The model under review builds one solid part; all positions refer to its coordinate system, in mm. A direction names the side the tool comes from. Round coordinates to 2 decimals unless told otherwise and drop trailing zeros. Loops run counter-clockwise (first coordinate to the right, second up) from the corner with the lowest first, then second, coordinate; pieces in that order, holes last. Notation, with made-up numbers: M -38,0 L -15,0 A17 cw -15,15 Z; hole C 52.25,-10.75 d2. An arc over 180 degrees is marked long. Answer as a JSON object with one key per item and string values. Group by question number.
Item 1: Consider section A-A (y = 20.5). Give the boundary of the cut face in (x, z), and give its area (3 significant figures).
Item 2: Consider section C-C (y = 10.75). Give the boundary of the cut face in (x, z), and give its area (3 significant figures).
Item 3: The part is to be moulded in two halves that separate along X. For faces 3 (the face through (-1, 23, 0)), 4 (the face through (19, 0, -7)), 5 (the face through (1, 23, 0)), 6 (the face through (19.394, 11.586, 12.365)), say which applies: +X half, -X half, draft (parallel to the pull), parting line (faces both ways), or undercut.
Item 4: Tool access review of faces 1 (the face through (0, 12, 0)), 2 (the face through (0, 25, 0)): name each direction out of +Z, -Z, +X, -X, +Y, -Y from which nothing blocks a thin tool from reaching the whole face with its end or side.
Item 5: To check wall thickness, follow line 1 (Z direction, x = -0.5, y = 16); line 2 (X direction, y = 11.9, z = 0); line 3 (Y direction, x = -1, z = 0). State the ranges of each line that lie inside material, in increasing order.
Item 6: Insertion check: P1, Ø1.3, axis at x = -2.5, z = -1.5, coming from the -Y side; P2, Ø8, axis at x = -11, y = 20, coming from the +Z side; P3, Ø5, axis at y = 15.5, z = -1.5, coming from the +X side. Each pin has a flat end and moves straight along its axis. Give the tip position at first contact, or say it passes through.
Item 7: Consider section B-B (y = 3.75). Give the boundary of the cut face in (x, z), and give its area (3 significant figures).
```python
from build123d import *

# Parameters (mm, degrees)
SKETCH1_R           = 23
BOSS_EXTRUDE1_DEPTH = 25
CUT_EXTRUDE1_DEPTH  = 23
SKETCH4_R           = 10
CUT_EXTRUDE2_DEPTH  = 12
CHAMFER1_SIZE       = 10
CHAMFER1_SIZE2      = 11.917535926
FILLET1_R           = 1.5
FILLET2_R           = 1


with BuildPart() as part:
    # Sketch1 → Boss-Extrude1 (new body)
    with BuildSketch(Plane(origin=(0, 0, 0), x_dir=(1, 0, 0), z_dir=(0, 1, 0))):
        with Locations(Location((0, 0, 0), (0, 0, 270))):
            Circle(SKETCH1_R)
    extrude(amount=BOSS_EXTRUDE1_DEPTH)

    # Sketch3 → Cut-Extrude1 (cut)
    with BuildSketch(Plane(origin=(0, 0, 0), x_dir=(-1, 0, 0), z_dir=(0, -1, 0))):
        with BuildLine():
            Line((-0.45, -3.067164815), (-0.45, 3.067164815))
            ThreePointArc((-0.45, 3.067164815), (-3.1, 0), (-0.45, -3.067164815))
        make_face()
        with BuildLine():
            ThreePointArc((3.1, 0), (2.345740821, 2.02669682), (0.45, 3.067164815))
            Line((0.45, 3.067164815), (0.45, -3.067164815))
            ThreePointArc((0.45, -3.067164815), (2.345740821, -2.02669682), (3.1, 0))
        make_face()
    extrude(amount=-CUT_EXTRUDE1_DEPTH, mode=Mode.SUBTRACT)

    # Sketch4 → Cut-Extrude2 (cut)
    with BuildSketch(Plane(origin=(0, 0, 0), x_dir=(-1, 0, 0), z_dir=(0, -1, 0))):
        with Locations(Location((0, 0, 0), (0, 0, 90))):
            Circle(SKETCH4_R)
    extrude(amount=-CUT_EXTRUDE2_DEPTH, mode=Mode.SUBTRACT)

    # Chamfer1
    chamfer1_edges = [part.edges().sort_by_distance(p)[0] for p in [
        (0, 0, 10),
    ]]
    chamfer1_side = [part.faces().sort_by_distance(p)[0] for p in [
        (0, 0, -22.349461761),
    ]]
    chamfer(chamfer1_edges, length=CHAMFER1_SIZE, length2=CHAMFER1_SIZE2, reference=chamfer1_side[0])

    # Fillet1
    fillet1_edges = [part.edges().sort_by_distance(p)[0] for p in [
        (0, 25, -23),
    ]]
    fillet(fillet1_edges, radius=FILLET1_R)

    # Sketch5 → Cut-Revolve1 (revolve, cut)
    with BuildSketch(Plane.XY):
        with BuildLine():
            Line((13, 25), (13, 23.5))
            ThreePointArc((13, 23.5), (14.60360392, 24.042792159), (16, 25))
            Line((16, 25), (13, 25))
        make_face()
    revolve(axis=Axis((13, 25, 0), (0, -1, 0)), mode=Mode.SUBTRACT)

    # Fillet2
    fillet2_edges = [part.edges().sort_by_distance(p)[0] for p in [
        (10, 25, 0),
    ]]
    fillet(fillet2_edges, radius=FILLET2_R)


solid = part.part
```
Geometry results:
{
 "1": {"outline": "C 0,0 d46; hole M -0.45,-3.07 L -0.45,3.07 A3.1 ccw Z; hole M 0.45,-3.07 A3.1 ccw 0.45,3.07 Z", "area": "1,640 mm^2"},
 "2": {"outline": "C 0,0 d46; hole C 0,0 d21.96", "area": "1,280 mm^2"},
 "3": {"face 3": "undercut", "face 4": "draft", "face 5": "undercut", "face 6": "parting line"},
 "4": {"face 1": "-Y", "face 2": "+Z, -Z, +X, -X, +Y"},
 "5": {"line 1": "z = -22.99 to -3.06, 3.06 to 22.99", "line 2": "x = -23 to -10.01, 10.01 to 23", "line 3": "y = 23 to 25"},
 "6": {"P1": "stops at y = 12", "P2": "stops at z = 21.91", "P3": "stops at x = 23"},
 "7": {"outline": "C 0,0 d46; hole C 0,0 d33.71", "area": "770 mm^2"}
}
